Can you work these out from the model? Positions are in its coordinate system, mm. A direction names the side the tool comes from. Coordinates: 2 decimals unless noted, no trailing zeros. Order: outer loops, then holes, each group sorted by start corner. A loop starts at its lowest first (then second) coordinate and runs counter-clockwise, first axis right, second up. Notation, with made-up numbers: (-5, -3) -> (46, -3) arc R10 ccw to (46, 5) -> close; hole circle Ø9 at (22, 79). An arc over 180 degrees is marked (long way). Answer in a Markdown table with one row per item.
```python
from build123d import *

# Parameters (mm, degrees)
ESBO_O1_W                = 152
ESBO_O1_H                = 164.64
RESSALTO_EXTRUS_O1_DEPTH = 4
FILETE1_R                = 3
RESSALTO_EXTRUS_O2_DEPTH = 4
FILETE2_R                = 3
FILETE3_R                = 1
CHANFRO1_SIZE            = 1.5
CHANFRO2_SIZE            = 1
ESBO_O3_R                = 2.1
CORTE_EXTRUS_O1_DEPTH    = 1


with BuildPart() as part:
    # Esboço1 → Ressalto-extrusão1 (new body)
    with BuildSketch(Plane.XY):
        Rectangle(ESBO_O1_W, ESBO_O1_H)
    extrude(amount=RESSALTO_EXTRUS_O1_DEPTH)

    # Filete1
    filete1_edges = [part.edges().sort_by_distance(p)[0] for p in [
        (76, -82.32, 2),
        (-76, -82.32, 2),
        (-76, 82.32, 2),
        (76, 82.32, 2),
    ]]
    fillet(filete1_edges, radius=FILETE1_R)

    # Esboço2 → Ressalto-extrusão2 (add)
    with BuildSketch(Plane(origin=(0, 0, 0), x_dir=(-1, 0, 0), z_dir=(0, 0, -1))):
        Polygon((-71.5, -73.32), (71.5, -73.32), (71.5, -40.35), (61, -40.35), (61, -35.35), (71.5, -35.35), (71.5, -21.68), (45, -21.68), (45, 56.32), (71.5, 56.32), (71.5, 77.82), (-71.5, 77.82), (-71.5, 56.32), (-45, 56.32), (-45, -21.68), (-71.5, -21.68), (-71.5, -35.35), (-61, -35.35), (-61, -40.35), (-71.5, -40.35), align=None)
    extrude(amount=RESSALTO_EXTRUS_O2_DEPTH)

    # Filete2
    filete2_edges = [part.edges().sort_by_distance(p)[0] for p in [
        (-71.5, 77.82, -2),
        (71.5, 77.82, -2),
        (45, 56.32, -2),
        (45, -21.68, -2),
        (71.5, -73.32, -2),
        (-71.5, -73.32, -2),
        (-45, -21.68, -2),
        (-45, 56.32, -2),
    ]]
    fillet(filete2_edges, radius=FILETE2_R)

    # Filete3
    filete3_edges = [part.edges().sort_by_distance(p)[0] for p in [
        (-71.5, 56.32, -2),
        (71.5, 56.32, -2),
        (71.5, -21.68, -2),
        (71.5, -35.35, -2),
        (61, -35.35, -2),
        (71.5, -40.35, -2),
        (-71.5, -40.35, -2),
        (-61, -35.35, -2),
        (-71.5, -35.35, -2),
        (-71.5, -21.68, -2),
    ]]
    fillet(filete3_edges, radius=FILETE3_R)

    # Chanfro1
    chanfro1_edges = [part.edges().sort_by_distance(p)[0] for p in [
        (-76, 0, 4),
        (0, 82.32, 4),
        (76, 0, 4),
        (0, -82.32, 4),
        (75.121320344, 81.441320344, 4),
        (75.121320344, -81.441320344, 4),
        (-75.121320344, -81.441320344, 4),
        (-75.121320344, 81.441320344, 4),
    ]]
    chamfer(chanfro1_edges, length=CHANFRO1_SIZE)

    # Chanfro2
    chanfro2_edges = [part.edges().sort_by_distance(p)[0] for p in [
        (71.5, 66.07, -4),
        (0, 77.82, -4),
        (45, 17.32, -4),
        (59.25, -21.68, -4),
        (0, -73.32, -4),
        (-71.5, -55.835, -4),
        (-45, 17.32, -4),
        (-59.25, 56.32, -4),
        (70.621320344, -72.441320344, -4),
        (-70.621320344, -72.441320344, -4),
        (-70.621320344, 76.941320344, -4),
        (70.621320344, 76.941320344, -4),
        (45.878679656, 55.441320344, -4),
        (45.878679656, -20.801320344, -4),
        (-45.878679656, -20.801320344, -4),
        (-45.878679656, 55.441320344, -4),
        (-65.75, -40.35, -4),
        (59.25, 56.32, -4),
        (71.5, -28.515, -4),
        (66.25, -35.35, -4),
        (61, -38.35, -4),
        (71.5, -55.835, -4),
        (-66.25, -35.35, -4),
        (-71.5, -28.515, -4),
        (-59.25, -21.68, -4),
        (-71.5, 66.07, -4),
        (71.207106781, -35.057106781, -4),
        (71.207106781, -21.972893219, -4),
        (71.207106781, 56.612893219, -4),
        (-71.207106781, 56.612893219, -4),
        (-71.207106781, -21.972893219, -4),
        (-71.207106781, -35.057106781, -4),
        (71.207106781, -40.642893219, -4),
        (-71.207106781, -40.642893219, -4),
        (-61.292893219, -35.642893219, -4),
        (61.292893219, -35.642893219, -4),
        (65.75, -40.35, -4),
        (-61, -38.35, -4),
    ]]
    chamfer(chanfro2_edges, length=CHANFRO2_SIZE)

    # Esboço3 → Corte-extrusão1 (cut)
    with BuildSketch(Plane(origin=(0, 0, 0), x_dir=(-1, 0, 0), z_dir=(0, 0, -1))):
        with Locations((-68, 48.32)):
            Circle(ESBO_O3_R)
        with Locations((-68, -11.68)):
            Circle(ESBO_O3_R)
        with Locations((-68, 18.32)):
            Circle(ESBO_O3_R)
        with Locations(Location((68, 18.32, 0), (0, 0, 180))):
            Circle(ESBO_O3_R)
        with Locations(Location((68, -11.68, 0), (0, 0, 180))):
            Circle(ESBO_O3_R)
        with Locations(Location((68, 48.32, 0), (0, 0, 180))):
            Circle(ESBO_O3_R)
    extrude(amount=-CORTE_EXTRUS_O1_DEPTH, mode=Mode.SUBTRACT)


solid = part.part
```
(1) Suppose I cut it at B-B (y = 18.32). Please give me the cut outline in (x, z), and give its area (3 significant figures).
Response values:
| item | result |
|---|---|
| outline | (-76, 0) -> (-70.1, 0) -> (-70.1, 1) -> (-65.9, 1) -> (-65.9, 0) -> (-45, 0) -> (-45, -3) -> (-44, -4) -> (44, -4) -> (45, -3) -> (45, 0) -> (65.9, 0) -> (65.9, 1) -> (70.1, 1) -> (70.1, 0) -> (76, 0) -> (76, 2.5) -> (74.5, 4) -> (-74.5, 4) -> (-76, 2.5) -> close |
| area | 956 mm2 |
(2) Suppose I cut it at D-D (x = -16). Please give me the cut outline in (y, z), and give its area (3 significant figures).
Response values:
| item | result |
|---|---|
| outline | (-82.32, 0) -> (-73.32, 0) -> (-73.32, -3) -> (-72.32, -4) -> (76.82, -4) -> (77.82, -3) -> (77.82, 0) -> (82.32, 0) -> (82.32, 2.5) -> (80.82, 4) -> (-80.82, 4) -> (-82.32, 2.5) -> close |
| area | 1,260 mm2 |
(3) On a 3-axis mill with a long thin cutter (end or side, diameter ignored), from which of +Z, -Z, +X, -X, +Y, -Y can I reach the whole of each face in a straight line? I mean faces 1 (the cylindrical face through (68.3, 50.4, 0.5)), 2 (the conical face through (-45.703, -21.028, -3.285)), 3 (the conical face through (45.703, 55.668, -3.285)). Say none if no direction works.
Response values:
| item | result |
|---|---|
| face 1 | -Z |
| face 2 | -Z, -X |
| face 3 | -Z, +X |
(4) Suppose I cut it at C-C (y = 37.5). Please give me the cut outline in (x, z), and give its area (3 significant figures).
Response values:
| item | result |
|---|---|
| outline | (-76, 0) -> (-45, 0) -> (-45, -3) -> (-44, -4) -> (44, -4) -> (45, -3) -> (45, 0) -> (76, 0) -> (76, 2.5) -> (74.5, 4) -> (-74.5, 4) -> (-76, 2.5) -> close |
| area | 965 mm2 |
(5) Will these pins go through, and if not, where does the flat tip stop? pin 1 Ø0.9 at (y, z) = (17.5, -2) entering from -X; pin 2 Ø0.9 at (y, z) = (-39, -1.5) entering from -X; pin 3 Ø0.9 at (x, z) = (-65, -1) entering from +Y.
Response values:
| item | result |
|---|---|
| pin 1 | x = -45 |
| pin 2 | x = -61 |
| pin 3 | y = 77.82 |
(6) Suppose I cut it at A-A (x = -55). Please give me the cut outline in (y, z), and give its area (3 significant figures).
Response values:
| item | result |
|---|---|
| outline | (-82.32, 0) -> (-73.32, 0) -> (-73.32, -3) -> (-72.32, -4) -> (-22.68, -4) -> (-21.68, -3) -> (-21.68, 0) -> (56.32, 0) -> (56.32, -3) -> (57.32, -4) -> (76.82, -4) -> (77.82, -3) -> (77.82, 0) -> (82.32, 0) -> (82.32, 2.5) -> (80.82, 4) -> (-80.82, 4) -> (-82.32, 2.5) -> close |
| area | 947 mm2 |
(7) I need wall thicknesses on line 1 (Y direction, x = -68, z = 0.3); line 2 (Z direction, x = 54.5, y = -0.5); line 3 (Y direction, x = -2.5, z = -0.75). Which ranges of each line are inside material? Lowest first, please. Write a range as [from, to].
Response values:
| item | result |
|---|---|
| line 1 | [-82.32, -13.78], [-9.58, 16.22], [20.42, 46.22], [50.42, 82.32] |
| line 2 | [0, 4] |
| line 3 | [-73.32, 77.82] |
